Input: part model. Units: mm. Frame: model coordinates. Face numbers are marked on the shaded views. A direction names the side the tool comes from. Give positions to 0.01 mm unless a question says otherwise; leave off trailing zeros. Write each loop counter-clockwise with the first axis right and the second up, starting at its lowest first coordinate (ties: lowest second). Pieces come first, ordered by that corner, then holes. Notation, with made-up numbers: (40, 11.25) - (57, 11.25) arc R6 ccw to (57, 15.25) - close; hole circle Ø6 at (18.25, 40.25). An arc over 180 degrees is marked (long way). Answer as CSV lines item,"result".
```python
from build123d import *

# Parameters (mm, degrees)
BOSS_EXTRUDE1_DEPTH = 20
CUT_EXTRUDE1_DEPTH  = 10
CUT_EXTRUDE3_DEPTH  = 20


with BuildPart() as part:
    # Sketch1 → Boss-Extrude1 (new body)
    with BuildSketch(Plane.XY):
        Polygon((0, 0), (15, 0), (15, 25), (-15, 25), (-15, 15), (-10, 15), align=None)
    extrude(amount=BOSS_EXTRUDE1_DEPTH)

    # Sketch2 → Cut-Extrude1 (cut)
    with BuildSketch(Plane.XY.offset(20)):
        Polygon((0, 0), (0, 25), (-15, 25), (-15, 15), (-10, 15), align=None)
    extrude(amount=-CUT_EXTRUDE1_DEPTH, mode=Mode.SUBTRACT)

    # Sketch3 → Cut-Extrude3 (cut)
    with BuildSketch(Plane.ZY):
        Polygon((10, 25), (20, 15), (20, 25), align=None)
    extrude(amount=-CUT_EXTRUDE3_DEPTH, mode=Mode.SUBTRACT)


solid = part.part
```
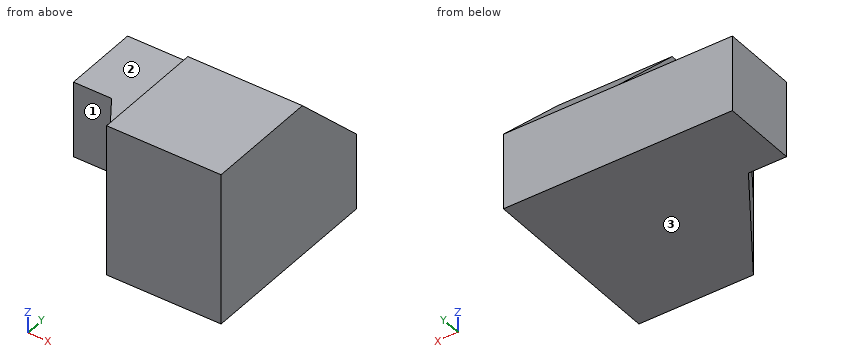
Item 1: Ray query, line 1 (Y direction, x = -10.75, z = 1.5); line 2 (Z direction, x = -5.5, y = 14.25); line 3 (X direction, y = 1.75, z = 11). Return the intervals inside material, ascending. Write a range as from..to.
The answers:
line 1,"15..25"
line 2,"0..10"
line 3,"0..15"
Item 2: Contact query for flat-ended pins moving along their axis: pin 1 (4.5 mm diameter, centred on x = -7, y = 8.5, fed in from +Z); pin 2 (5 mm diameter, centred on x = 0, z = 16, fed in from +Y); pin 3 (5 mm diameter, centred on x = 3, y = 22, fed in from +Z); pin 4 (1 mm diameter, centred on x = 7, y = 15, fed in from -Z). Output: stop coordinate, or through.
The answers:
pin 1,"z = 10"
pin 2,"y = 21.5"
pin 3,"z = 15.5"
pin 4,"z = 0"
Item 3: Cut plane C-C on z = 6.5. Return the cut outline in (x, y).
The answers:
outline,"(-15, 15) - (-10, 15) - (0, 0) - (15, 0) - (15, 25) - (-15, 25) - close"
Item 4: Reachability of the marked faces 1, 2 and 3 from +Z, -Z, +X, -X, +Y, -Y: full face, straight path, thin tool, end or side. Return the list, or none.
The answers:
face 1,"+Z, -Z, -X, -Y"
face 2,"+Z, -X, +Y, -Y"
face 3,"-Z, +X, -X, +Y, -Y"
Item 5: Cut plane D-D on z = 14. Return the cut outline in (x, y), plus the area to 3 significant figures.
The answers:
outline,"(0, 0) - (15, 0) - (15, 21) - (0, 21) - close"
area,"315 mm²"
Item 6: Cut plane A-A on x = 10.25. Return the cut outline in (y, z).
The answers:
outline,"(0, 0) - (25, 0) - (25, 10) - (15, 20) - (0, 20) - close"
Item 7: Cut plane B-B on y = 15.5. Return the cut outline in (x, z), plus the area to 4 significant figures.
The answers:
outline,"(-15, 0) - (15, 0) - (15, 19.5) - (0, 19.5) - (0, 10) - (-15, 10) - close"
area,"442.5 mm²"
